Source: CAD feature listing. Evaluate the final solid. Frame: model axes, mm. Face numbers are marked on the shaded views. A direction names the side the tool comes from. Coordinates: 2 decimals unless noted, no trailing zeros. Order: outer loops, then holes, each group sorted by start corner. A loop starts at its lowest first (then second) coordinate and runs counter-clockwise, first axis right, second up. Notation, with made-up numbers: (54.25, 76.5) -> (85.25, 76.5) arc R31 ccw to (85.25, 108.5) -> close; hole circle Ø1 at (16.5, 52). An arc over 180 degrees is marked (long way). Put each result on its own line as item: value.
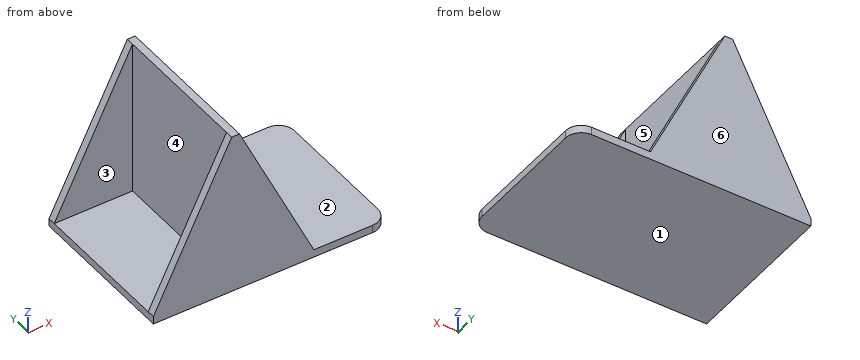
from build123d import *

# Parameters (mm, degrees)
F0_W     = 48.26
F0_H     = 50.8
F0_W_2   = 25.4
F0_W_3   = 2.54
F1_DEPTH = 2.54
F2_DEPTH = 50.8
F4_DEPTH = 2.54
F6_DEPTH = 2.54
F7_R     = 5.08


with BuildPart() as f1:
    # F0 (on Top) → F1 (new body)
    with BuildSketch(Plane.XY):
        with Locations((29.726995, 6.723735)):
            Rectangle(F0_W, F0_H)
        with Locations((-9.643005, 6.723735)):
            Rectangle(F0_W_2, F0_H)
        with Locations((4.326995, 6.723735)):
            Rectangle(F0_W_3, F0_H)
    extrude(amount=-F1_DEPTH)

    # F0 (on Top) → F2 (join)
    with BuildSketch(Plane.XY):
        with Locations((4.326995, 6.723735)):
            Rectangle(F0_W_3, F0_H)
    extrude(amount=F2_DEPTH)

    # F3 (on face) → F4 (join)
    with BuildSketch(Plane.XZ.offset(18.676265)):
        Polygon((3.056995, 50.8), (-22.343005, 0), (3.056995, 0), align=None)
        Polygon((29.726995, 0), (5.596995, 50.8), (5.596995, 0), align=None)
    extrude(amount=-F4_DEPTH)

    # F5 (on face) → F6 (join)
    with BuildSketch(Plane(origin=(0, 32.123735, 0), x_dir=(-1, 0, 0), z_dir=(0, 1, 0))):
        Polygon((22.343005, 0), (-3.056995, 50.8), (-3.056995, 0), align=None)
        Polygon((-5.596995, 0), (-5.596995, 50.8), (-29.726995, 0), align=None)
    extrude(amount=-F6_DEPTH)

    # F7
    f7_edges = [f1.edges().sort_by_distance(p)[0] for p in [
        (53.856995, -18.676265, -1.27),
        (53.856995, 32.123735, -1.27),
    ]]
    fillet(f7_edges, radius=F7_R)


solid = f1.part
1. Cut plane A-A on y = 1.5. Output: boundary loops of the cut face in (x, z), plus the area to 3 significant figures.
Numbers:
outline: (-22.34, -2.54) -> (53.86, -2.54) -> (53.86, 0) -> (5.6, 0) -> (5.6, 50.8) -> (3.06, 50.8) -> (3.06, 0) -> (-22.34, 0) -> close
area: 323 mm2
2. Cut plane B-B on z = 12. Output: boundary loops of the cut face in (x, y).
Numbers:
outline: (-16.34, -18.68) -> (24.03, -18.68) -> (24.03, -16.14) -> (5.6, -16.14) -> (5.6, 29.58) -> (24.03, 29.58) -> (24.03, 32.12) -> (-16.34, 32.12) -> (-16.34, 29.58) -> (3.06, 29.58) -> (3.06, -16.14) -> (-16.34, -16.14) -> close
3. First-contact query: pin 1 (6 mm diameter, centred on y = 22.5, z = 16.5, fed in from -X); pin 2 (1 mm diameter, centred on y = -12, z = 39, fed in from +X); pin 3 (24 mm diameter, centred on x = 28.5, y = 5, fed in from +Z). Flat tips, straight axial feed; report the tip coordinate or a pass-through.
Numbers:
pin 1: stops at x = 3.06
pin 2: stops at x = 5.6
pin 3: stops at z = 0
4. Ray query, line 1 along Y through (x, z) = (1, 11); line 2 along Z through (x, y) = (14, -14); line 3 along X through (y, z) = (-14.5, 45.5). Return the intervals inside material, ascending.
Numbers:
line 1: y = -18.68 to -16.14, 29.58 to 32.12
line 2: z = -2.54 to 0
line 3: x = 3.06 to 5.6
5. Cut plane D-D on z = 26.5. Output: boundary loops of the cut face in (x, y).
Numbers:
outline: (-9.09, -18.68) -> (17.14, -18.68) -> (17.14, -16.14) -> (5.6, -16.14) -> (5.6, 29.58) -> (17.14, 29.58) -> (17.14, 32.12) -> (-9.09, 32.12) -> (-9.09, 29.58) -> (3.06, 29.58) -> (3.06, -16.14) -> (-9.09, -16.14) -> close
6. Set-up query: the marked faces 4, 5 and 6. Return all of +Z, -Z, +X, -X, +Y, -Y with unobstructed straight access to the full face (end or side cutting, diameter ignored); none if empty.
Numbers:
face 4: +Z, -X
face 5: +Z, +X
face 6: +Z, -Z, +X, -X, +Y
7. Cut plane C-C on x = -1. Output: boundary loops of the cut face in (y, z).
Numbers:
outline: (-18.68, -2.54) -> (32.12, -2.54) -> (32.12, 42.69) -> (29.58, 42.69) -> (29.58, 0) -> (-16.14, 0) -> (-16.14, 42.69) -> (-18.68, 42.69) -> close
8. Pull-direction query (Z, two-part tool) for the marked faces 1, 2 and 3; classes: pulls with the +Z half, pulls with the -Z half, needs draft (parallel to the pull), parting line crosses it, or undercut.
Numbers:
face 1: pulls with the -Z half
face 2: pulls with the +Z half
face 3: needs draft
